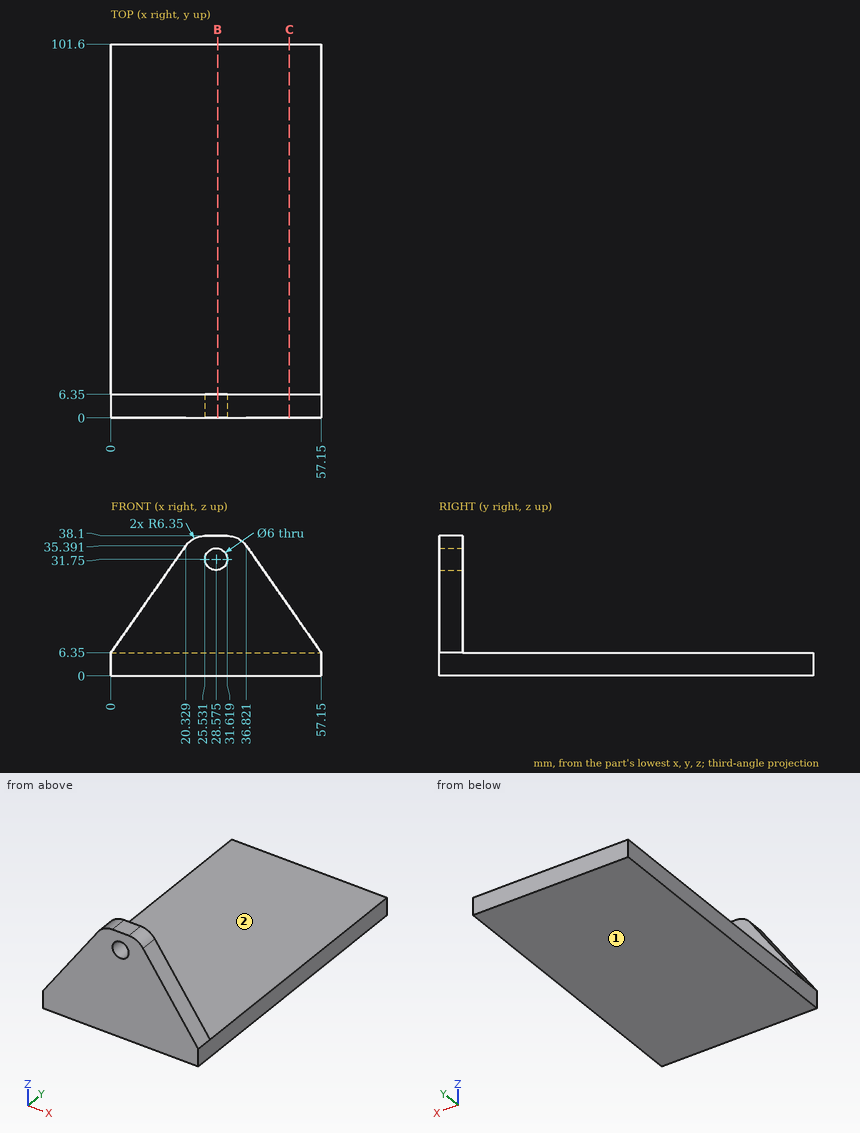
Design review of the part shown in the three views and the two pictorial views. Dimensions are in mm from the part's minimum x, y and z. A direction names the side the tool comes from. Round coordinates to 2 decimals unless told otherwise and drop trailing zeros. Loops run counter-clockwise (first coordinate to the right, second up) from the corner with the lowest first, then second, coordinate; pieces in that order, holes last. Notation, with made-up numbers: M 11,56 L 64,56 A31 cw 64,88 Z; hole C 46,44 d5. An arc over 180 degrees is marked long. Put each result on its own line as item: value.
Q1. To check wall thickness, follow L1, parallel to Y at x = 12.5, z = 7.5. State the ranges of the line that lie inside material, in increasing order.
Result set:
L1: y = 0 to 6.35
Q2. For pin 1 (1.5 mm diameter, centred on x = 26.5, y = 65, fed in from +Z); pin 2 (7 mm diameter, centred on x = 28.575, z = 31.75, fed in from +Y), all flat-tipped, find the tip position at first contact; note any pin that passes through.
Result set:
pin 1: stops at z = 6.35
pin 2: stops at y = 6.35
Q3. Machinability: for the marked faces 1 and 2, which of the approach directions +Z, -Z, +X, -X, +Y, -Y give a long, thin tool a straight path to every point of the face, cutting with its end or side? Answer none if there is none.
Result set:
face 1: -Z, +X, -X, +Y, -Y
face 2: +Z, +X, -X, +Y
Q4. Consider section B-B, the plane x = 29. Give the boundary of the cut face in (y, z).
Result set:
outline: M 0,0 L 101.6,0 L 101.6,6.35 L 6.35,6.35 L 6.35,28.78 L 0,28.78 Z; M 0,34.72 L 6.35,34.72 L 6.35,38.1 L 0,38.1 Z
Q5. Consider section C-C, the plane x = 48.5. Give the boundary of the cut face in (y, z).
Result set:
outline: M 0,0 L 101.6,0 L 101.6,6.35 L 6.35,6.35 L 6.35,18.71 L 0,18.71 Z
